Can you work these out from the model? Positions are in its coordinate system, mm. A direction names the side the tool comes from. Give positions to 0.01 mm unless a question says otherwise; leave off trailing zeros. Loops run counter-clockwise (first coordinate to the right, second up) from the corner with the lowest first, then second, coordinate; pieces in that order, holes last. Notation, with made-up numbers: (20, 11.25) - (66, 11.25) arc R21 cw to (66, 30.25) - close; hole circle Ø10 at (43.5, 63). An arc over 180 degrees is marked (long way). Answer as a JSON object with one key per item and string values.
```python
from build123d import *

# Parameters (mm, degrees)
SKETCH_1_W      = 30
SKETCH_1_H      = 60
SKETCH_1_R      = 1.7
SKETCH_1_W_2    = 20
SKETCH_1_H_2    = 40.5
SKETCH_1_R_2    = 10
SKETCH_1_R_3    = 4.15
EXTRUDE_1_DEPTH = 8
FILLET_1_R      = 5


with BuildPart() as part:
    # Эскиз1 → Бобышка-Вытянуть1 (new body)
    # profile 1 of 3: a face of its own
    with BuildSketch(Plane.XY):
        with Locations((0, 69.5)):
            Rectangle(SKETCH_1_W, SKETCH_1_H)
        with Locations((-5, 44)):
            Circle(SKETCH_1_R, mode=Mode.SUBTRACT)
        with Locations((5, 95)):
            Circle(SKETCH_1_R, mode=Mode.SUBTRACT)
        with Locations((-5, 95)):
            Circle(SKETCH_1_R, mode=Mode.SUBTRACT)
        with Locations((5, 44)):
            Circle(SKETCH_1_R, mode=Mode.SUBTRACT)
        with Locations((0, 69.5)):
            Rectangle(SKETCH_1_W_2, SKETCH_1_H_2, mode=Mode.SUBTRACT)
    # profile 2 of 3: a face of its own
    with BuildSketch(Plane.XY):
        Circle(SKETCH_1_R_2)
        Circle(SKETCH_1_R_3, mode=Mode.SUBTRACT)
    # profile 3 of 3: a face of its own
    with BuildSketch(Plane.XY):
        with BuildLine():
            Line((-10, 39.5), (-10, 0))
            ThreePointArc((-10, 0), (0, 10), (10, 0))
            Line((10, 0), (10, 39.5))
            Line((10, 39.5), (-10, 39.5))
        make_face()
    extrude(amount=EXTRUDE_1_DEPTH)

    # Скругление1
    fillet_1_edges = [part.edges().sort_by_distance(p)[0] for p in [
        (15, 39.5, 4),
        (-15, 39.5, 4),
        (-15, 99.5, 4),
        (15, 99.5, 4),
    ]]
    fillet(fillet_1_edges, radius=FILLET_1_R - 0.0001)  # a hair under: the kernel refuses the full size


solid = part.part
```
1) Which directions (+Z, -Z, +X, -X, +Y, -Y) give clear straight access to the entire face, cutting with the end or side of a thin tool? Please do faces 1 (the flat face through (10, 19, 4)), 2 (the flat face through (0, 99.5, 4)), 3 (the flat face through (-10, 20, 4)), 4 (the flat face through (15, 69, 4)), 5 (the flat face through (10, 69, 4)).
Check sheet entries:
{"face 1": "+Z, -Z, +X, -Y", "face 2": "+Z, -Z, +X, -X, +Y", "face 3": "+Z, -Z, -X, -Y", "face 4": "+Z, -Z, +X, +Y, -Y", "face 5": "+Z, -Z"}
2) I'm going to push flat-ended pins straight in: P1, Ø2.5, axis at y = 28.5, z = 5.5, coming from the +X side; P2, Ø1, axis at x = -2.5, z = 4, coming from the -Y side; P3, Ø1.5, axis at x = -8.5, z = 6, coming from the -Y side. Where does each tip first touch, or does it pass through?
Check sheet entries:
{"P1": "x = 10", "P2": "y = -9.8", "P3": "y = -6.32"}
3) Imagine slicing it at A-A on x = 0. Write out the boundary of the cut face in (y, z), and give its area (3 significant figures).
Check sheet entries:
{"outline": "(-10, 0) - (-4.15, 0) - (-4.15, 8) - (-10, 8) - close; (4.15, 0) - (49.25, 0) - (49.25, 8) - (4.15, 8) - close; (89.75, 0) - (99.5, 0) - (99.5, 8) - (89.75, 8) - close", "area": "486 mm2"}
4) I need wall thicknesses on L1, parallel to Y at x = 0, z = 3; L2, parallel to X at y = 95.5, z = 5.75; L3, parallel to Y at x = 6, z = 1.5. Which ranges of each line are inside material? Lowest first, please.
Check sheet entries:
{"L1": "-10 to -4.15, 4.15 to 49.25, 89.75 to 99.5", "L2": "-14.9 to -6.62, -3.38 to 3.38, 6.62 to 14.9", "L3": "-8 to 42.63, 45.37 to 49.25, 89.75 to 93.63, 96.37 to 99.5"}
5) Imagine slicing it at C-C on y = 1. Write out the boundary of the cut face in (x, z), and give its area (3 significant figures).
Check sheet entries:
{"outline": "(-10, 0) - (-4.03, 0) - (-4.03, 8) - (-10, 8) - close; (4.03, 0) - (10, 0) - (10, 8) - (4.03, 8) - close", "area": "95.6 mm2"}
6) Imagine slicing it at D-D on z = 5.25. Give the number of separate pieces and of enclosed holes in the cut face, and give its area (3 significant figures).
Check sheet entries:
{"separate pieces": "1", "enclosed holes": "6", "area": "1,830 mm2"}
7) If we mould it in two halves opening along X, with no side actions, what happens to faces 6 (the cylindrical face through (-5.37, 93.34, 3.94)), 7 (the cylindrical face through (-13.57, 98, 4.06)), 8 (the flat face through (0, 46, 8)), 9 (the cylindrical face through (4.63, 93.34, 3.94))? For each: released by +X, released by -X, zero draft, split by the parting line, or undercut.
Check sheet entries:
{"face 6": "undercut", "face 7": "released by -X", "face 8": "zero draft", "face 9": "undercut"}
8) Imagine slicing it at B-B on x = -8. Write out the boundary of the cut face in (y, z), and give its area (3 significant figures).
Check sheet entries:
{"outline": "(-6, 0) - (49.25, 0) - (49.25, 8) - (-6, 8) - close; (89.75, 0) - (99.5, 0) - (99.5, 8) - (89.75, 8) - close", "area": "520 mm2"}
